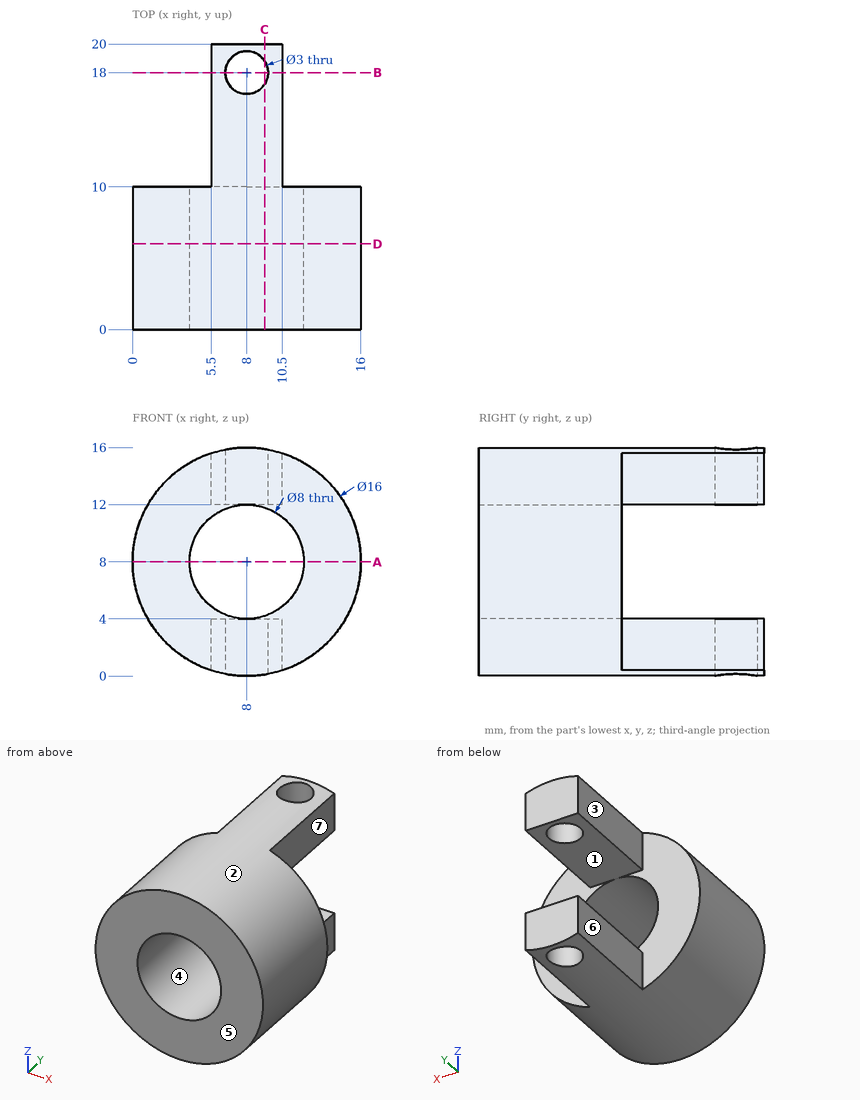
Print and shaded views of the part. All mm, measured from the part's lowest x, y and z. A direction names the side the tool comes from. Coordinates: 2 decimals unless noted, no trailing zeros. Order: outer loops, then holes, each group sorted by start corner. A loop starts at its lowest first (then second) coordinate and runs counter-clockwise, first axis right, second up.
Item 1: Mould opens along Z. For the marked faces 1, 2, 3 and 4 say: released by +Z, released by -Z, zero draft, split by the parting line, or undercut.
Filled in:
face 1: undercut
face 2: split by the parting line
face 3: zero draft
face 4: undercut
Item 2: Saw through at C-C on x = 9.25. List the corners of the cut face in (y, z), then the cut area to 3 significant figures.
Filled in:
outline: (0, 0.1) - (17.17, 0.1) - (17.17, 4) - (10, 4) - (10, 4.2) - (0, 4.2) - close; (0, 11.8) - (10, 11.8) - (10, 12) - (17.17, 12) - (17.17, 15.9) - (0, 15.9) - close; (18.83, 0.1) - (20, 0.1) - (20, 4) - (18.83, 4) - close; (18.83, 12) - (20, 12) - (20, 15.9) - (18.83, 15.9) - close
area: 147 mm2
Item 3: Drill centre lines: L1, parallel to Y at x = 12, z = 9.75; L2, parallel to Z at x = 5, y = 3.5; L3, parallel to Z at x = 8.5, y = 13.5. Where is each one in solid material? Low to high.
Filled in:
L1: y = 0 to 10
L2: z = 0.58 to 5.35, 10.65 to 15.42
L3: z = 0.02 to 4, 12 to 15.98
Item 4: Saw through at B-B on y = 18. List the corners of the cut face in (x, z).
Filled in:
outline: (5.5, 0.4) arc R8 ccw to (6.5, 0.14) - (6.5, 4) - (5.5, 4) - close; (5.5, 12) - (6.5, 12) - (6.5, 15.86) arc R8 ccw to (5.5, 15.6) - close; (9.5, 0.14) arc R8 ccw to (10.5, 0.4) - (10.5, 4) - (9.5, 4) - close; (9.5, 12) - (10.5, 12) - (10.5, 15.6) arc R8 ccw to (9.5, 15.86) - close
Item 5: Tool access for the marked faces 5, 6 and 7: list every direction of +Z, -Z, +X, -X, +Y, -Y with a clear straight run to the whole face (end or side of a thin tool).
Filled in:
face 5: +Z, -Z, +X, -X, -Y
face 6: +Z, -Z, -X, +Y
face 7: +Z, -Z, +X, +Y
Item 6: Drop flat-ended pins along their axis: pin 1 Ø4 at (x, z) = (14, 8) entering from +Y; pin 2 Ø3 at (y, z) = (17, 2.5) entering from -X; pin 3 Ø4 at (y, z) = (4, 5.5) entering from -X. Give the stop position or say it passes through.
Filled in:
pin 1: stops at y = 10
pin 2: stops at x = 5.5
pin 3: stops at x = 0.02
Item 7: Saw through at A-A on z = 8. List the corners of the cut face in (x, y), then the cut area to 3 significant figures.
Filled in:
outline: (0, 0) - (4, 0) - (4, 10) - (0, 10) - close; (12, 0) - (16, 0) - (16, 10) - (12, 10) - close
area: 80.0 mm2
Item 8: Saw through at D-D on y = 6. List the corners of the cut face in (x, z).
Filled in:
outline: circle Ø16 at (8, 8); hole circle Ø8 at (8, 8)
